Drawing for the job (mm, zero at the part's lowest x, y, z). Round coordinates to 2 decimals unless told otherwise and drop trailing zeros. Loops run counter-clockwise (first coordinate to the right, second up) from the corner with the lowest first, then second, coordinate; pieces in that order, holes last. Notation, with made-up numbers: M -19.75,49.5 L 0.25,49.5 A22 cw 0.25,57.5 Z; hole C -21.5,72.5 d2. An arc over 180 degrees is marked long. Answer in a Markdown table with one row per item.
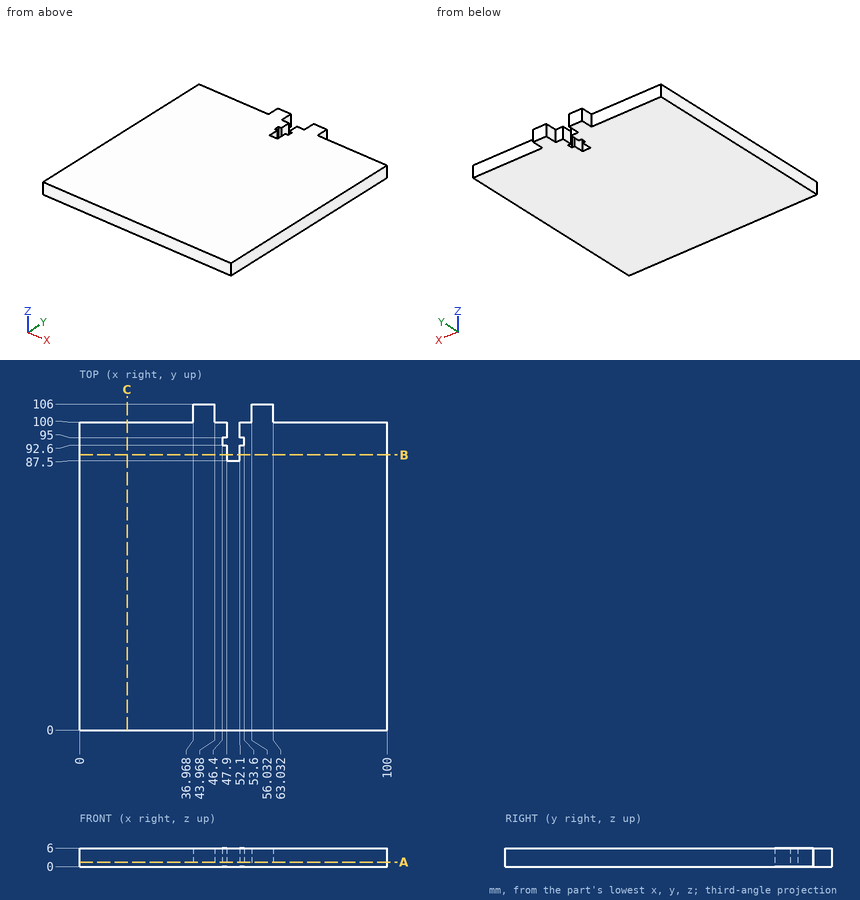
1. Saw through at C-C (x = 15.5). Write the cut outline in (y, z), and give its area (3 significant figures).
Verdict:
| item | result |
|---|---|
| outline | M 0,0 L 100,0 L 100,6 L 0,6 Z |
| area | 600 mm² |
2. Saw through at A-A (z = 1.45). Write the cut outline in (x, y), and give its area (3 significant figures).
Verdict:
| item | result |
|---|---|
| outline | M 0,0 L 100,0 L 100,100 L 63.03,100 L 63.03,106 L 56.03,106 L 56.03,100 L 52.1,100 L 52.1,95 L 53.6,95 L 53.6,92.6 L 52.1,92.6 L 52.1,87.5 L 47.9,87.5 L 47.9,92.6 L 46.4,92.6 L 46.4,95 L 47.9,95 L 47.9,100 L 43.97,100 L 43.97,106 L 36.97,106 L 36.97,100 L 0,100 Z |
| area | 10,000 mm² |
3. Saw through at B-B (y = 89.5). Write the cut outline in (x, z).
Verdict:
| item | result |
|---|---|
| outline | M 0,0 L 47.9,0 L 47.9,6 L 0,6 Z; M 52.1,0 L 100,0 L 100,6 L 52.1,6 Z |
4. Pin check, flat tips, straight feed: pin 1 (1.7 mm diameter, centred on x = 53, z = 4, fed in from -Y); pin 2 (3 mm diameter, centred on y = 103.5, z = 2.5, fed in from +X); pin 3 (3 mm diameter, centred on x = 21.5, z = 3, fed in from +Y); pin 4 (1.8 mm diameter, centred on y = 103, z = 3.5, fed in from -X). Stop position of each tip, or through.
Verdict:
| item | result |
|---|---|
| pin 1 | stops at y = 0 |
| pin 2 | stops at x = 63.03 |
| pin 3 | stops at y = 100 |
| pin 4 | stops at x = 36.97 |
5. Wall check: probe 1 along X at (y, z) = (96.5, 4.45); probe 2 along Y at (x, z) = (13, 0.4). Give the ranges that are in metal, low to high.
Verdict:
| item | result |
|---|---|
| probe 1 | x = 0 to 47.9, 52.1 to 100 |
| probe 2 | y = 0 to 100 |
